from build123d import *

# Parameters (mm, degrees)
SKETCH1_W               = 76.2
SKETCH1_H               = 304.8
BOSS_EXTRUDE1_DEPTH     = 1.5875
SKETCH2_R               = 6.35
BOSS_EXTRUDE2_DEPTH     = 304.8
CUT_EXTRUDE1_DEPTH      = 72.4535
CUT_EXTRUDE1_DEPTH_BACK = 72.4535
SKETCH3_W               = 22.233491501
SKETCH3_H               = 25.4
SKETCH3_W_2             = 25.169990379
SKETCH3_W_3             = 20.176908814
SKETCH4_R               = 5.08
CUT_EXTRUDE2_DEPTH      = 332.781682839


with BuildPart() as part:
    # Sketch1 → Boss-Extrude1 (new body)
    with BuildSketch(Plane.XY):
        with Locations((-92.340618933, 15.386782554)):
            Rectangle(SKETCH1_W, SKETCH1_H)
    extrude(amount=BOSS_EXTRUDE1_DEPTH)

    # Sketch2 → Boss-Extrude2 (add)
    with BuildSketch(Plane(origin=(0, 167.786782554, 0), x_dir=(1, 0, 0), z_dir=(0, 1, 0))):
        with Locations((-54.240618933, -6.35)):
            Circle(SKETCH2_R)
    extrude(amount=-BOSS_EXTRUDE2_DEPTH)

    # Sketch3 → Cut-Extrude1 (cut, two sides: drawn at the far end of the back side and taken through both)
    with BuildSketch(Plane.XY.offset(1.5875).offset(-CUT_EXTRUDE1_DEPTH_BACK)):
        with Locations((-49.473873183, 129.686782554)):
            Rectangle(SKETCH3_W, SKETCH3_H)
        with Locations((-49.473873183, 78.886782554)):
            Rectangle(SKETCH3_W, SKETCH3_H)
        with Locations((-49.473873183, 28.086782554)):
            Rectangle(SKETCH3_W, SKETCH3_H)
        with Locations((-49.473873183, -22.713217446)):
            Rectangle(SKETCH3_W, SKETCH3_H)
        with Locations((-48.005623744, -73.513217446)):
            Rectangle(SKETCH3_W_2, SKETCH3_H)
        with Locations((-50.502164526, -124.313217446)):
            Rectangle(SKETCH3_W_3, SKETCH3_H)
    extrude(amount=CUT_EXTRUDE1_DEPTH + CUT_EXTRUDE1_DEPTH_BACK, mode=Mode.SUBTRACT)

    # Sketch4 → Cut-Extrude2 (cut, through all)
    with BuildSketch(Plane(origin=(0, 167.786782554, 0), x_dir=(1, 0, 0), z_dir=(0, 1, 0))):
        with Locations(Location((-54.240618933, -6.35, 0), (0, 0, 270))):
            Circle(SKETCH4_R)
    extrude(amount=-CUT_EXTRUDE2_DEPTH, mode=Mode.SUBTRACT)


solid = part.part
The listing builds one solid part. Answer for the finished solid, in the listing's coordinates (mm). A direction names the side the tool comes from. Round coordinates to 2 decimals unless told otherwise and drop trailing zeros. Write each loop counter-clockwise with the first axis right and the second up, starting at its lowest first coordinate (ties: lowest second). Pieces come first, ordered by that corner, then holes. Notation, with made-up numbers: M 46,81 L 97,81 A24 cw 97,93 Z; hole C -32.5,-27.75 d6. An arc over 180 degrees is marked long. Write each question's results on one line, items separated by ' | '. Start each with the question number.
(1) Find the intervals of material crossed by line 1 (Y direction, x = -52.5, z = 1); line 2 (X direction, y = 6.5, z = 6.35); line 3 (Z direction, x = -112, y = -28.5), in increasing order.
(2) Each of these flat-tipped pins is pushed along its axis until it touches: P1, Ø0.5, axis at y = 126, z = 1, coming from the +X side; P2, Ø3, axis at x = -63, y = 74, coming from the +Z side; P3, Ø6.5, axis at x = -51.5, z = 9, coming from the -Y side. Where does it stop, or does it pass through?
(3) The part is cut by section A-A, the plane y = 95. Write down the section's boundary in (x, z), and give its area (3 significant figures).
(4) The part is cut by section B-B, the plane z = 6.35. Give the number of separate pieces and of enclosed holes in the cut face, and give its area (3 significant figures).
(5) The part is cut by section C-C, the plane x = -118. Write down the section's boundary in (y, z).
(6) For faces 4 (the cylindrical face through (-49.204, 53.665, 5.689)), 5 (the flat face through (-59, -86.213, 3)), determine the directions among +Z, -Z, +X, -X, +Y, -Y from which every point of the face is accessible in a straight line to the end or side of a thin tool.
(7) Determine the mould class of faces 1 (the flat face through (-59, -10.013, 3)), 2 (the cylindrical face through (-49.204, 155.265, 5.689)), 3 (the flat face through (-59, -111.613, 3)) for opening direction Y: +Y half, -Y half, draft (parallel to the pull), parting line (faces both ways), or undercut.
Worked answers:
1) line 1: y = -111.61 to -86.21, -60.81 to -35.41, -10.01 to 15.39, 40.79 to 66.19, 91.59 to 116.99, 142.39 to 167.79 | line 2: x = -60.59 to -59.32, -49.16 to -47.89 | line 3: z = 0 to 1.59
2) P1: stops at x = -60.59 | P2: stops at z = 1.59 | P3: stops at y = -111.61
3) outline: M -130.44,0 L -54.24,0 A6.35 ccw long -58.44,1.59 L -130.44,1.59 Z; hole C -54.24,6.35 d10.16 | area: 162 mm²
4) separate pieces: 12 | enclosed holes: 0 | area: 387 mm²
5) outline: M -137.01,0 L 167.79,0 L 167.79,1.59 L -137.01,1.59 Z
6) face 4: +Y, -Y | face 5: +Z, -Z, +X
7) face 1: undercut | face 2: draft | face 3: -Y half
